Source: CAD feature listing. Evaluate the final solid. Frame: model axes, mm. Face numbers are marked on the shaded views. A direction names the side the tool comes from. Give positions to 0.01 mm unless a question says otherwise; leave off trailing zeros. Loops run counter-clockwise (first coordinate to the right, second up) from the corner with the lowest first, then second, coordinate; pieces in that order, holes last. Notation, with made-up numbers: M 26.5,11 L 31.5,11 A16 ccw 31.5,17 Z; hole C -8,78.5 d11. An arc over 180 degrees is marked long. Answer in a Markdown table with one row per item.
```python
from build123d import *

# Parameters (mm, degrees)
BOSS_EXTRU_1_DEPTH      = 11
BOSS_EXTRU_2_DEPTH      = 26
BOSS_EXTRU_3_DEPTH      = 11
ESQUISSE4_R             = 11
BOSS_EXTRU_4_DEPTH      = 2
ESQUISSE5_R             = 2.5
BOSS_EXTRU_5_DEPTH      = 22
ESQUISSE6_W             = 5.798316384
ESQUISSE6_H             = 1
ENL_V_MAT_EXTRU_1_DEPTH = 18
TROU_TARAUD_M31_D       = 2.5
TROU_TARAUD_M31_DEPTH   = 7
TROU_TARAUD_M31_TIP     = 0.751075774
ESQUISSE9_W             = 6.3
ESQUISSE9_H             = 4.75
BOSS_EXTRU_6_DEPTH      = 2.3
ESQUISSE10_R            = 0.2025
BOSS_EXTRU_7_DEPTH      = 10
ESQUISSE11_R            = 0.55
BOSS_EXTRU_8_DEPTH      = 8


with BuildPart() as part:
    # Esquisse1 → Boss.-Extru.1 (new body)
    with BuildSketch(Plane.XY):
        Polygon((17, 21), (21, 17), (21, -17), (17, -21), (-17, -21), (-21, -17), (-21, 17), (-17, 21), align=None)
    extrude(amount=BOSS_EXTRU_1_DEPTH)

    # Esquisse2 → Boss.-Extru.2 (add)
    with BuildSketch(Plane(origin=(0, 0, 0), x_dir=(-1, 0, 0), z_dir=(0, 0, -1))):
        Polygon((-16, 21), (16, 21), (21, 16), (21, -16), (16, -21), (-16, -21), (-21, -16), (-21, 16), align=None)
    extrude(amount=BOSS_EXTRU_2_DEPTH)

    # Esquisse3 → Boss.-Extru.3 (add)
    with BuildSketch(Plane(origin=(0, 0, -26), x_dir=(-1, 0, 0), z_dir=(0, 0, -1))):
        Polygon((-17, 21), (-21, 17), (-21, -17), (-17, -21), (17, -21), (21, -17), (21, 17), (17, 21), align=None)
    extrude(amount=BOSS_EXTRU_3_DEPTH)

    # Esquisse4 → Boss.-Extru.4 (add)
    with BuildSketch(Plane(origin=(0, 0, -37), x_dir=(-1, 0, 0), z_dir=(0, 0, -1))):
        Circle(ESQUISSE4_R)
    extrude(amount=BOSS_EXTRU_4_DEPTH)

    # Esquisse5 → Boss.-Extru.5 (add)
    with BuildSketch(Plane(origin=(0, 0, -39), x_dir=(-1, 0, 0), z_dir=(0, 0, -1))):
        Circle(ESQUISSE5_R)
    extrude(amount=BOSS_EXTRU_5_DEPTH)

    # Esquisse6 → Enlèv. mat.-Extru.1 (cut)
    with BuildSketch(Plane(origin=(0, 0, -61), x_dir=(-1, 0, 0), z_dir=(0, 0, -1))):
        with Locations((0, 2.5)):
            Rectangle(ESQUISSE6_W, ESQUISSE6_H)
    extrude(amount=-ENL_V_MAT_EXTRU_1_DEPTH, mode=Mode.SUBTRACT)

    # Trou taraudé M31
    with Locations(Plane(origin=(0, 0, -37), x_dir=(-1, 0, 0), z_dir=(0, 0, -1))):
        with Locations((-15.5, 15.5), (15.5, 15.5), (15.5, -15.5), (-15.5, -15.5)):
            Hole(TROU_TARAUD_M31_D / 2, depth=TROU_TARAUD_M31_DEPTH)
            with Locations((0, 0, -(TROU_TARAUD_M31_DEPTH + TROU_TARAUD_M31_TIP / 2))):  # 118° drill point
                Cone(0, TROU_TARAUD_M31_D / 2, TROU_TARAUD_M31_TIP, mode=Mode.SUBTRACT)

    # Esquisse9 → Boss.-Extru.6 (add)
    with BuildSketch(Plane.XZ.offset(21)):
        with Locations((0, 6.925)):
            Rectangle(ESQUISSE9_W, ESQUISSE9_H)
    extrude(amount=BOSS_EXTRU_6_DEPTH)

    # Esquisse10 → Boss.-Extru.7 (add)
    with BuildSketch(Plane.XZ.offset(23.3)):
        with Locations((-2.25, 6.925)):
            Circle(ESQUISSE10_R)
        with Locations((-0.75, 6.925)):
            Circle(ESQUISSE10_R)
        with Locations((0.75, 6.925)):
            Circle(ESQUISSE10_R)
        with Locations((2.25, 6.925)):
            Circle(ESQUISSE10_R)
    extrude(amount=BOSS_EXTRU_7_DEPTH)

    # Esquisse11 → Boss.-Extru.8 (add)
    with BuildSketch(Plane.XZ.offset(23.3)):
        with Locations((-2.25, 6.925)):
            Circle(ESQUISSE11_R)
        with Locations((-0.75, 6.925)):
            Circle(ESQUISSE11_R)
        with Locations((0.75, 6.925)):
            Circle(ESQUISSE11_R)
        with Locations((2.25, 6.925)):
            Circle(ESQUISSE11_R)
    extrude(amount=BOSS_EXTRU_8_DEPTH)


solid = part.part
```
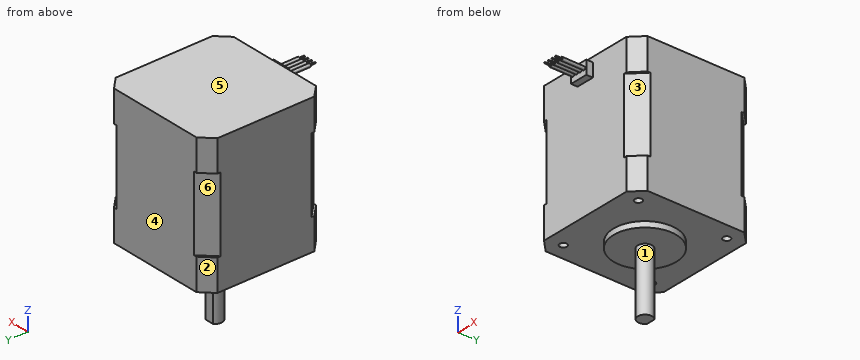
1) Material intervals for L1, parallel to Y at x = -15.5, z = -31.75; L2, parallel to Y at x = 15, z = -31, sorted ascending.
Reply:
| item | result |
|---|---|
| L1 | y = -21 to -16.75, -14.25 to 14.25, 16.75 to 21 |
| L2 | y = -21 to -16.65, -14.35 to 14.35, 16.65 to 21 |
2) Section D-D, the plane y = -27.5. Return loops of the section in (x, z) (3 decimals).
Reply:
| item | result |
|---|---|
| outline | C -2.25,6.925 d1.1; C -0.75,6.925 d1.1; C 0.75,6.925 d1.1; C 2.25,6.925 d1.1 |
3) Pull-direction query (Z, two-part tool) for the marked faces 4, 5 and 6; classes: released by +Z, released by -Z, zero draft, split by the parting line, or undercut.
Reply:
| item | result |
|---|---|
| face 4 | zero draft |
| face 5 | released by +Z |
| face 6 | undercut |
4) Section C-C, the plane x = 12. Return loops of the section in (y, z).
Reply:
| item | result |
|---|---|
| outline | M -21,-37 L 21,-37 L 21,11 L -21,11 Z |
5) Set-up query: the marked faces 1, 2 and 3. Return all of +Z, -Z, +X, -X, +Y, -Y with unobstructed straight access to the full face (end or side cutting, diameter ignored); none if empty.
Reply:
| item | result |
|---|---|
| face 1 | -Z |
| face 2 | +Z, -Z, -X, +Y |
| face 3 | +X, -Y |
6) Section B-B, the plane z = -27. Return loops of the section in (x, y).
Reply:
| item | result |
|---|---|
| outline | M -21,-17 L -17,-21 L 17,-21 L 21,-17 L 21,17 L 17,21 L -17,21 L -21,17 Z |
7) Pin query (flat end, axial travel): pin 1 Ø1.2 at (y, z) = (-22, 6) entering from +X; pin 2 Ø8 at (y, z) = (-6, -45.5) entering from -X; pin 3 Ø4 at (x, y) = (-19, -19.5) entering from -Z; pin 4 Ø4 at (x, z) = (0.5, 8) entering from -Y. Return the tip coordinate at first contact, or that it passes through.
Reply:
| item | result |
|---|---|
| pin 1 | stops at x = 3.15 |
| pin 2 | stops at x = -1.5 |
| pin 3 | stops at z = -37 |
| pin 4 | stops at y = -33.3 |
8) Section A-A, the plane y = 0. Return loops of the section in (x, z).
Reply:
| item | result |
|---|---|
| outline | M -21,-37 L -11,-37 L -11,-39 L -2.5,-39 L -2.5,-61 L 2.5,-61 L 2.5,-39 L 11,-39 L 11,-37 L 21,-37 L 21,11 L -21,11 Z |
